Autodesk Inventor part; units mm, degrees
ref_plane "YZ Plane" through (0, 0, 0) normal (1, 0, 0) x (0, 1, 0)
ref_plane "XZ Plane" through (0, 0, 0) normal (0, 1, 0) x (-1, 0, 0)
ref_plane "XY Plane" through (0, 0, 0) normal (0, 0, 1) x (1, 0, 0)
sketch "スケッチ1" plane through (0, 0, 0) normal (0, 0, 1) x (1, 0, 0)
  circle A0 centre (0, 0) radius 10.5 construction
  line L0 (0, 10.5) -> (-162.5, 10.5) construction
  line L1 (-162.5, 10.5) -> (-162.5, -10.5) construction
  line L2 (-162.5, -10.5) -> (0, -10.5) construction
  circle A1 centre (-157.5, 0) radius 1.55 construction
  line L3 (-147.5, 2.5) -> (-32.5, 2.5) construction
  line L4 (-32.5, 2.5) -> (-32.5, -2.5) construction
  line L5 (-32.5, -2.5) -> (-147.5, -2.5) construction
  line L6 (-147.5, -2.5) -> (-147.5, 2.5) construction
  line L7 (-90, 2.5) -> (-90, -2.5) construction
  circle A2 centre (-22.5, 0) radius 1.55 construction
  line L8 (-12, 21.3027) -> (-12, -27.3903) construction
  line L9 (-32.45, 2.55) -> (-147.55, 2.55) construction
  line L10 (-147.55, 2.55) -> (-147.55, -2.55) construction
  line L11 (-147.55, -2.55) -> (-32.45, -2.55) construction
  line L12 (-32.45, -2.55) -> (-32.45, 2.55) construction
  circle A3 centre (-146.5, 2.55) radius 1.05 construction
  line L13 (-147.5, 0) -> (-90, 0) construction
  line L14 (-147.55, 2.55) -> (-147.55, -2.55) construction
  arc A4 (-145.45, 2.55) -> (-147.55, 2.55) centre (-146.5, 2.55) ccw construction
  line L15 (-145.45, 2.55) -> (-34.55, 2.55) construction
  arc A5 (-32.45, 2.55) -> (-34.55, 2.55) centre (-33.5, 2.55) ccw construction
  line L16 (-32.45, 2.55) -> (-32.45, -2.55) construction
  arc A6 (-147.55, -2.55) -> (-145.45, -2.55) centre (-146.5, -2.55) ccw construction
  line L17 (-145.45, -2.55) -> (-34.55, -2.55) construction
  arc A7 (-34.55, -2.55) -> (-32.45, -2.55) centre (-33.5, -2.55) ccw construction
  circle A8 centre (0, 8.5) radius 1.35
  circle A9 centre (0, 0) radius 5.05
  circle A10 centre (-8.5, 0) radius 1.35
  circle A11 centre (0, -8.5) radius 1.35
  circle A12 centre (8.5, 0) radius 1.35
  line L18 (-162.5, 4.8006) -> (-162.5, -4.8006) construction
  line L19 (-162.5, 4.8006) -> (-22.5, 10.5) construction
  line L20 (-22.5, 10.5) -> (0, 10.5) construction
  line L21 (-162.5, -4.8006) -> (-22.5, -10.5) construction
  line L22 (-22.5, -10.5) -> (0, -10.5) construction
  arc A13 (0, -10.5) -> (0, 10.5) centre (0, 0) ccw construction
  circle A14 centre (-157.5, 0) radius 5 construction
  circle A15 centre (-21.5, 0) radius 1.55
  circle A16 centre (-46.5, 0) radius 1.55
  line L23 (-17.5, -2.5) -> (-50.5, -2.5) construction
  line L24 (-50.5, -2.5) -> (-50.5, 2.5) construction
  line L25 (-50.5, 2.5) -> (-17.5, 2.5) construction
  line L26 (-17.5, 2.5) -> (-17.5, -2.5) construction
  line L27 (-27.5, -2.5) -> (-40.5, -2.5) construction
  line L28 (-40.5, -2.5) -> (-40.5, 2.5) construction
  line L29 (-40.5, 2.5) -> (-27.5, 2.5) construction
  line L30 (-27.5, 2.5) -> (-27.5, -2.5) construction
  line L31 (-27.45, -2.55) -> (-40.55, -2.55)
  line L32 (-40.55, -2.55) -> (-40.55, 2.55)
  line L33 (-40.55, 2.55) -> (-27.45, 2.55)
  line L34 (-27.45, 2.55) -> (-27.45, -2.55)
  circle A17 centre (-28.5, -2.55) radius 1.05
  circle A18 centre (-28.5, 2.55) radius 1.05
  circle A19 centre (-39.5, -2.55) radius 1.05
  circle A20 centre (-39.5, 2.55) radius 1.05
  line L35 (-50.5, 2.5) -> (-50.5, -2.5)
  line L36 (-50.5, -2.5) -> (-16.9113, -10.5)
  line L37 (-50.5, 2.5) -> (-16.9113, 10.5)
  arc A21 (0, -10.5) -> (0, 10.5) centre (0, 0) ccw
  line L38 (-16.9113, 10.5) -> (0, 10.5)
  line L39 (0, -10.5) -> (-16.9113, -10.5)
  circle A22 centre (-39.5, 2.55) radius 2.5 construction
  circle A23 centre (0, 0) radius 16 construction
  circle A24 centre (0, 0) radius 21 construction
  line L40 (-21, 19.3585) -> (-21, -28.09) construction
  point P0 (-162.5, 0)
  point P1 (-17.5, 0)
  dimension "d9" = 2.1
  dimension "d29" = 2.1
  dimension "d0" = 162.5
  dimension "d1" = 3.1
  dimension "d2" = 21
  dimension "d3" = 10
  dimension "d4" = 5
  dimension "d5" = 12
  dimension "d6" = 135
  dimension "d7" = 5
  dimension "d8" = 0.05
  dimension "d10" = 2.7
  dimension "d11" = 8.5
  dimension "d12" = 10.1
  dimension "d15" = 360
  dimension "d20" = 3.1
  dimension "d21" = 5
  dimension "d22" = 4
  dimension "d23" = 5
  dimension "d24" = 25
  dimension "d26" = 10
  dimension "d27" = 4
  dimension "d28" = 10
  dimension "d30" = 0.05
  dimension "d32" = 5
  dimension "d33" = 32
  dimension "d34" = 5
extrude "押し出し1" add sketch "スケッチ1" along normal blind 2
fillet "フィレット2" radius 2 2 edges at (-50.5, 2.5, 1) (-50.5, -2.5, 1)
equation "\"d2\" = d2_1"
equation "\"d3\" = d3_1"
equation "\"d4\" = d4_1"
equation "\"d6\" = d6_1"
equation "\"d21\" = d4"
equation "\"d27\" = d22"
equation "\"d28\" = d26"
properties part number "前腕_メインフレーム_1_1" material "GFRP"
Verification items for the finished model (mm, model axes). A direction names the side the tool comes from. Coordinates: 2 decimals unless noted, no trailing zeros. Order: outer loops, then holes, each group sorted by start corner. A loop starts at its lowest first (then second) coordinate and runs counter-clockwise, first axis right, second up.
Item 1: Section check A-A, the plane z = 1.3. Give the number of separate pieces and of enclosed holes in the cut face, then the cut area to 3 significant figures.
Filled in:
separate pieces: 1
enclosed holes: 8
area: 772 mm2
Item 2: Material ranges on L1, parallel to Y at x = 0, z = 0.55; L2, parallel to X at y = 2.5, z = 1.3; L3, parallel to Y at x = -8.5, z = 0.6, recorded low to high.
Filled in:
L1: y = -10.5 to -9.85, -7.15 to -5.05, 5.05 to 7.15, 9.85 to 10.5
L2: x = -49.73 to -40.55, -27.45 to -4.39, 4.39 to 10.2
L3: y = -10.5 to -1.35, 1.35 to 10.5
Item 3: Depth check by flat-ended pin: pin 1 (1 mm diameter, centred on x = -34, z = 0.5, fed in from -Y); pin 2 (1 mm diameter, centred on y = -1, z = 1, fed in from +X). Enter the tip coordinate at first touch or a pass-through.
Filled in:
pin 1: stops at y = -6.55
pin 2: stops at x = 10.49
Item 4: Access from +Z, -Z, +X, -X, +Y, -Y to the whole of each face (thin tool, end or side, straight path). Record for faces 5 (the face through (-14, 0, 2)), 6 (the face through (-40.55, 0, 1)).
Filled in:
face 5: +Z, +X, -X, +Y, -Y
face 6: +Z, -Z
Item 5: Section check B-B, the plane x = -46.5. Enter the section's corners in (y, z), then the cut area to 3 significant figures.
Filled in:
outline: (-3.45, 0) - (-1.55, 0) - (-1.55, 2) - (-3.45, 2) - close; (1.55, 0) - (3.45, 0) - (3.45, 2) - (1.55, 2) - close
area: 7.61 mm2
Item 6: Release check for a two-part mould opening along Y. For faces 1 (the face through (-9, 10.5, 1)), 2 (the face through (-8, -10.5, 1)), 3 (the face through (10.5, 0.2, 1)), 4 (the face through (4.817, -1.517, 0.986)) record: +Y half, -Y half, draft (parallel to the pull), parting line (faces both ways), or undercut.
Filled in:
face 1: +Y half
face 2: -Y half
face 3: parting line
face 4: undercut
Item 7: Section check D-D, the plane y = -6. Enter the section's corners in (x, z), then the cut area to 3 significant figures.
Filled in:
outline: (-35.8, 0) - (8.62, 0) - (8.62, 2) - (-35.8, 2) - close
area: 88.8 mm2
Item 8: Section check C-C, the plane y = 8.5. Enter the section's corners in (x, z), then the cut area to 3 significant figures.
Filled in:
outline: (-25.31, 0) - (-1.35, 0) - (-1.35, 2) - (-25.31, 2) - close; (1.35, 0) - (6.16, 0) - (6.16, 2) - (1.35, 2) - close
area: 57.5 mm2
